Source: CAD feature listing. Evaluate the final solid. Frame: model axes, mm. Face numbers are marked on the shaded views. A direction names the side the tool comes from. Coordinates: 2 decimals unless noted, no trailing zeros. Order: outer loops, then holes, each group sorted by start corner. A loop starts at its lowest first (then second) coordinate and runs counter-clockwise, first axis right, second up. Notation, with made-up numbers: (-22.5, -10.5) - (29.5, -10.5) arc R21 cw to (29.5, 26.5) - close; hole circle Ø9 at (-7, -1). An arc over 180 degrees is marked (long way). One line per question, with ' | ' between items. Start each with the question number.
(1) Section D-D (x = 123). Return the cut outline in (y, z).
(2) Section B-B (x = 12.7). Return the cut outline in (y, z), then the cut area to 3 significant figures.
(3) Section A-A (z = -19.05). Return the cut outline in (x, y).
(4) Draft query along X for the marked faces 1, 2, 3 and 4. Return one class per face: +X half, -X half, draft (parallel to the pull), parting line (faces both ways), or undercut.
(5) Access query for the marked faces 5 and 6. Directions: +Z, -Z, +X, -X, +Y, -Y. A direction counts if a zero-diameter tool reaches every point of the face in a straight line with its end or side. Return the directions, or none.
(6) Section C-C (z = -30). Return the cut outline in (x, y).
(7) Contact query for flat-ended pins moving along their axis: P1, Ø8, axis at x = 38.5, z = -16, coming from the +Y side; P2, Ø8, axis at x = 76.25, y = 63.49, coming from the -Z side; P3, Ø1, axis at y = 14, z = -12.5, coming from the -X side; P4, Ø5, axis at x = 53, y = 60, coming from the +Z side. Output: stop coordinate, or through.
(8) Line query: line 1 along X through (y, z) = (9, -19.05); line 2 along Z through (x, y) = (139.7, 9.75); line 3 along Z through (x, y) = (80, 21.5). Output: solid intervals per line, ascending.
from build123d import *

# Parameters (mm, degrees)
SKETCH1_W                                = 152.4
SKETCH1_H                                = 38.1
BASEPLATE_DEPTH                          = 12.7
VERTBOSS_DEPTH                           = 12.7
F_9_32_0_28125_DIAMETER_HOLE1_D          = 7.14375
CBORE_FOR_1_4_HEX_HEAD_BOLT1_D           = 6.7564
CBORE_FOR_1_4_HEX_HEAD_BOLT1_CBORE_D     = 19.05
CBORE_FOR_1_4_HEX_HEAD_BOLT1_CBORE_DEPTH = 4.7752
SKETCH11_W                               = 38
SKETCH11_H                               = 3.17
BOTTOMSLOT_DEPTH                         = 178.43624207
FILLET1_R                                = 6.35
FILLET2_R                                = 3.17


with BuildPart() as part:
    # Sketch1 → BasePlate (new body)
    with BuildSketch(Plane(origin=(0, 0, 0), x_dir=(1, 0, 0), z_dir=(0, 1, 0))):
        with Locations((76.2, 19.05)):
            Rectangle(SKETCH1_W, SKETCH1_H)
    extrude(amount=BASEPLATE_DEPTH)

    # Sketch3 → VertBoss (add)
    with BuildSketch(Plane.XY):
        with BuildLine():
            Line((57.2, 0), (57.2, 63.5))
            ThreePointArc((57.2, 63.5), (76.2, 82.5), (95.2, 63.5))
            Line((95.2, 63.5), (95.2, 0))
            Line((95.2, 0), (57.2, 0))
        make_face()
    extrude(amount=-VERTBOSS_DEPTH)

    # 9/32 (0.28125) Diameter Hole1 (through all)
    with Locations(Plane(origin=(0, 12.7, 0), x_dir=(1, 0, 0), z_dir=(0, 1, 0))):
        with Locations((139.7, 19.05), (12.7, 19.05)):
            Hole(F_9_32_0_28125_DIAMETER_HOLE1_D / 2)

    # CBORE for 1/4 Hex Head Bolt1 (through all)
    with Locations(Plane.XY):
        with Locations((76.24706856, 63.487087048)):
            CounterBoreHole(CBORE_FOR_1_4_HEX_HEAD_BOLT1_D / 2, CBORE_FOR_1_4_HEX_HEAD_BOLT1_CBORE_D / 2, CBORE_FOR_1_4_HEX_HEAD_BOLT1_CBORE_DEPTH)

    # Sketch11 → BottomSlot (cut, through all)
    with BuildSketch(Plane.XY):
        with Locations((76.2, 1.585)):
            Rectangle(SKETCH11_W, SKETCH11_H)
    extrude(amount=-BOTTOMSLOT_DEPTH, mode=Mode.SUBTRACT)

    # Fillet1
    # the kernel refuses this fillet: 6.35 mm, written as the material it adds along each edge
    with BuildSketch(Plane(origin=(95.2, 3.17, 0), x_dir=(-1, 0, 0), z_dir=(0, 0, -1))) as fillet1_piece_1:
        with BuildLine():
            CenterArc((5.49637153, -6.35), FILLET1_R, 90, 59.947892244)
            Line((0, -3.17), (0, 0))
            Line((0, 0), (5.49637153, 0))
        make_face()
    extrude(amount=38.1)
    with BuildSketch(Plane(origin=(57.2, 3.17, 0), x_dir=(0, -1, 0), z_dir=(0, 0, -1))) as fillet1_piece_2:
        with BuildLine():
            CenterArc((6.35, -5.49637153), FILLET1_R, 120.052107756, 59.947892244)
            Line((0, -5.49637153), (0, 0))
            Line((0, 0), (3.17, 0))
        make_face()
    extrude(amount=38.1)
    # the kernel refuses this fillet: 6.35 mm, written as the material it takes off along each edge
    with BuildSketch(Plane(origin=(0, -15.875, -38.1), x_dir=(0, 0, 1), z_dir=(0, 1, 0)), Plane(origin=(0, -15.875, 0), x_dir=(1, 0, 0), z_dir=(0, 1, 0))) as fillet1_2_piece_1:
        with BuildLine():
            CenterArc((FILLET1_R, FILLET1_R), FILLET1_R, 180, 90)
            Line((0, FILLET1_R), (0, 0))
            Line((0, 0), (FILLET1_R, 0))
        make_face()
    extrude(amount=44.45, mode=Mode.SUBTRACT)
    with BuildSketch(Plane(origin=(152.4, -15.875, -38.1), x_dir=(0, 0, 1), z_dir=(0, 1, 0)), Plane(origin=(152.4, -15.875, 0), x_dir=(-1, 0, 0), z_dir=(0, 1, 0))) as fillet1_2_piece_2:
        with BuildLine():
            CenterArc((FILLET1_R, -FILLET1_R), FILLET1_R, 90, 90)
            Line((0, -FILLET1_R), (0, 0))
            Line((0, 0), (FILLET1_R, 0))
        make_face()
    extrude(amount=44.45, mode=Mode.SUBTRACT)

    # Fillet2
    fillet2_edges = [part.edges().sort_by_distance(p)[0] for p in [
        (120.625, 12.7, 0),
        (57.2, 38.1, -12.7),
        (95.2, 38.1, -12.7),
        (57.2, 38.1, 0),
        (95.2, 38.1, 0),
        (76.2, 82.5, 0),
        (57.2, 12.7, -6.35),
        (76.2, 82.5, -12.7),
        (95.2, 12.7, -6.35),
        (76.2, 12.7, -12.7),
        (0, 12.7, -19.05),
        (76.2, 12.7, -38.1),
        (31.775, 12.7, 0),
        (152.4, 12.7, -19.05),
        (150.540128061, 12.7, -1.859871939),
        (150.540128061, 12.7, -36.240128061),
        (1.859871939, 12.7, -1.859871939),
        (1.859871939, 12.7, -36.240128061),
    ]]
    fillet(fillet2_edges, radius=FILLET2_R)


solid = part.part
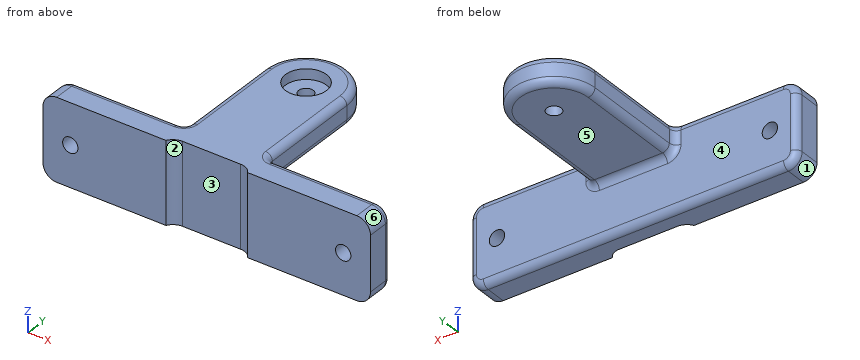
Response values:
1) outline: (0, -38.1) - (9.53, -38.1) arc R3.17 ccw to (12.7, -34.93) - (12.7, -3.17) arc R3.17 ccw to (9.53, 0) - (0, 0) - close
2) outline: (0, -38.1) - (9.53, -38.1) arc R3.17 ccw to (12.7, -34.93) - (12.7, -22.62) - (0, -22.62) - close; (0, -15.48) - (12.7, -15.48) - (12.7, -3.17) arc R3.17 ccw to (9.53, 0) - (0, 0) - close | area: 389 mm²
3) outline: (0, 0) - (9.13, 0) - (9.13, 12.7) - (3.17, 12.7) arc R3.17 ccw to (0, 9.53) - close; (16.27, 0) - (57.2, 0) arc R6.35 cw to (62.7, 3.17) - (89.7, 3.17) arc R6.35 cw to (95.2, 0) - (136.13, 0) - (136.13, 12.7) - (16.27, 12.7) - close; (143.27, 0) - (152.4, 0) - (152.4, 9.53) arc R3.17 ccw to (149.23, 12.7) - (143.27, 12.7) - close
4) face 1: -X half | face 2: undercut | face 3: undercut | face 4: draft
5) face 5: -Z, +X, -X, +Y | face 6: +Z, +X, +Y, -Y
6) outline: (0, 0) - (57.2, 0) arc R6.35 cw to (62.7, 3.17) - (89.7, 3.17) arc R6.35 cw to (95.2, 0) - (152.4, 0) - (152.4, 9.53) arc R3.17 ccw to (149.23, 12.7) - (3.17, 12.7) arc R3.17 ccw to (0, 9.53) - close
7) P1: stops at y = 12.7 | P2: stops at z = -12.7 | P3: stops at x = 57.22 | P4: passes through
8) line 1: x = 0 to 9.13, 16.27 to 136.13, 143.27 to 152.4 | line 2: z = -38.09 to -22.62, -15.48 to -0.01 | line 3: z = -12.7 to 0
